from build123d import *

# Parameters (mm, degrees)
SKETCH1_W           = 24
SKETCH1_H           = 24
SKETCH1_R           = 0.75
BOSS_EXTRUDE1_DEPTH = 5
FILLET1_R           = 5
CUT_EXTRUDE1_DEPTH  = 5


with BuildPart() as part:
    # Sketch1 → Boss-Extrude1 (new body)
    with BuildSketch(Plane.XY):
        Rectangle(SKETCH1_W, SKETCH1_H)
        with Locations((0, -9)):
            Circle(SKETCH1_R, mode=Mode.SUBTRACT)
        with Locations((-7.5, -1.5)):
            Circle(SKETCH1_R, mode=Mode.SUBTRACT)
        with Locations((7.5, -1.5)):
            Circle(SKETCH1_R, mode=Mode.SUBTRACT)
    extrude(amount=BOSS_EXTRUDE1_DEPTH)

    # Fillet1
    fillet1_edges = [part.edges().sort_by_distance(p)[0] for p in [
        (-12, 12, 2.5),
        (12, 12, 2.5),
    ]]
    fillet(fillet1_edges, radius=FILLET1_R)

    # Sketch2 → Cut-Extrude1 (cut)
    with BuildSketch(Plane.XY.offset(5)):
        Polygon((-10, -12), (-10, -10.5), (-11, -10.5), (-11, -8), (-10, -8), (-10, -7), (-6, -7), (-6, -8), (-5, -8), (-5, -10.5), (-6, -10.5), (-6, -12), align=None)
    cut_extrude1 = extrude(amount=-CUT_EXTRUDE1_DEPTH, mode=Mode.SUBTRACT)

    # Mirror1: Cut-Extrude1 across plane
    add(cut_extrude1.mirror(Plane(origin=(0, 0, 0), x_dir=(0, 0, 1), z_dir=(1, 0, 0))), mode=Mode.SUBTRACT)


solid = part.part
Read the model definition and answer for the solid it produces. Units are mm, in the model's axes. A direction names the side the tool comes from. Round coordinates to 2 decimals unless told otherwise and drop trailing zeros. Order: outer loops, then holes, each group sorted by start corner. A loop starts at its lowest first (then second) coordinate and runs counter-clockwise, first axis right, second up.
1) For faces 1 (the face through (-5.5, -10.5, 2.5)), 2 (the face through (10, 11, 3)), 3 (the face through (10, -11, 3)), determine the directions among +Z, -Z, +X, -X, +Y, -Y from which every point of the face is accessible in a straight line to the end or side of a thin tool.
2) The part is cut by section B-B on x = 0. Write down the section's boundary in (y, z), plus the area to 4 significant figures.
3) The part is cut by section A-A on y = -9. Write down the section's boundary in (x, z), plus the area to 3 significant figures.
4) The part is cut by section C-C on z = 3.5. Give the number of separate pieces and of enclosed holes in the cut face, plus the area to 3 significant figures.
5) The mould has two halves that part along X. Classify faces 4 (the face through (-8, -7, 3)), 5 (the face through (11, -12, 2)), 6 (the face through (12, -3, 2)): released by +X, released by -X, zero draft, split by the parting line, or undercut.
6) Flat-ended cylindrical pins translate along their axes: pin 1 (1.7 mm diameter, centred on x = 7.5, y = -1.5, fed in from -Z); pin 2 (1.1 mm diameter, centred on x = -10.5, z = 1.5, fed in from +Y); pin 3 (1.5 mm diameter, centred on x = 9, z = 4, fed in from -Y); pin 4 (1.2 mm diameter, centred on x = 0, y = -9, fed in from -Z). Find the tip coordinate at first contact, or state that the pin passes through.
7) The part is cut by section D-D on y = -1.5. Write down the section's boundary in (x, z), plus the area to 3 significant figures.
8) Straight lines are drawn through the part: L1, parallel to Y at x = 0, z = 1.05; L2, parallel to Y at x = -5.5, z = 3.65; L3, parallel to X at y = 10.5, z = 0.4. For each, find the intervals that lie inside material, in ascending order.
Resolved:
1. face 1: +Z, -Z
1. face 2: +Z, -Z, +X, +Y
1. face 3: +Z, -Z, -Y
2. outline: (-12, 0) - (-9.75, 0) - (-9.75, 5) - (-12, 5) - close; (-8.25, 0) - (12, 0) - (12, 5) - (-8.25, 5) - close
2. area: 112.5 mm2
3. outline: (-12, 0) - (-11, 0) - (-11, 5) - (-12, 5) - close; (-5, 0) - (-0.75, 0) - (-0.75, 5) - (-5, 5) - close; (0.75, 0) - (5, 0) - (5, 5) - (0.75, 5) - close; (11, 0) - (12, 0) - (12, 5) - (11, 5) - close
3. area: 52.5 mm2
4. separate pieces: 1
4. enclosed holes: 3
4. area: 510 mm2
5. face 4: undercut
5. face 5: zero draft
5. face 6: released by +X
6. pin 1: stops at z = 0
6. pin 2: stops at y = 11.04
6. pin 3: stops at y = -7
6. pin 4: passes through
7. outline: (-12, 0) - (-8.25, 0) - (-8.25, 5) - (-12, 5) - close; (-6.75, 0) - (6.75, 0) - (6.75, 5) - (-6.75, 5) - close; (8.25, 0) - (12, 0) - (12, 5) - (8.25, 5) - close
7. area: 105 mm2
8. L1: y = -12 to -9.75, -8.25 to 12
8. L2: y = -12 to -10.5, -8 to 12
8. L3: x = -10.57 to 10.57
